from build123d import *

# Parameters (mm, degrees)
F0_W      = 25
F0_H      = 11
F1_DEPTH  = 10
F2_R      = 8
F3_DEPTH  = 6
F4_R      = 6
F5_DEPTH  = 4.2
F6_W      = 11
F6_H      = 10
F7_DEPTH  = 2
F8_W      = 11
F8_H      = 10
F9_DEPTH  = 2
F10_R     = 5
F11_R     = 1.75
F12_DEPTH = 25
F9_FACE_W = 19
F9_FACE_H = 10
F13_DEPTH = 10
F14_R     = 8.137493
F15_DEPTH = 4.5
F17_DEPTH = 7
F18_R     = 4.5
F19_DEPTH = 25


with BuildPart() as f1:
    # F0 (on Top) → F1 (new body)
    with BuildSketch(Plane.XY):
        with Locations((12.5, 5.5)):
            Rectangle(F0_W, F0_H)
    extrude(amount=F1_DEPTH)

    # F2 (on face) → F3 (cut)
    with BuildSketch(Plane.XZ):
        with Locations((12.5, 10)):
            Circle(F2_R)
    extrude(amount=-F3_DEPTH, mode=Mode.SUBTRACT)

    # F4 (on face) → F5 (cut)
    with BuildSketch(Plane.XZ.offset(-6)):
        with Locations((12.5, 10)):
            Circle(F4_R)
    extrude(amount=-F5_DEPTH, mode=Mode.SUBTRACT)

    # F6 (on face) → F7 (join)
    with BuildSketch(Plane(origin=(0, 0, 0), x_dir=(0, -1, 0), z_dir=(-1, 0, 0))):
        with Locations((-5.5, 5)):
            Rectangle(F6_W, F6_H)
    extrude(amount=F7_DEPTH)

    # F8 (on face) → F9 (join)
    with BuildSketch(Plane.YZ.offset(25)):
        with Locations((5.5, 5)):
            Rectangle(F8_W, F8_H)
    extrude(amount=F9_DEPTH)

    # F10
    f10_edges = [f1.edges().sort_by_distance(p)[0] for p in [
        (27, 11, 5),
        (27, 0, 5),
        (-2, 11, 5),
        (-2, 0, 5),
    ]]
    fillet(f10_edges, radius=F10_R)

    # F11 (on face) → F12 (cut)
    with BuildSketch(Plane.XY.offset(10)):
        with Locations((0.75, 6.25)):
            Circle(F11_R)
        with Locations((24.25, 6.25)):
            Circle(F11_R)
    extrude(amount=-F12_DEPTH, mode=Mode.SUBTRACT)

    # F9_face (on face) → F13 (join)
    with BuildSketch(Plane(origin=(12.5, 11, 5), x_dir=(-1, 0, 0), z_dir=(0, 1, 0))):
        Rectangle(F9_FACE_W, F9_FACE_H)
    extrude(amount=F13_DEPTH)

    # F14 (on face) → F15 (cut)
    with BuildSketch(Plane.XZ.offset(-10.2)):
        with Locations((12.5, 10)):
            Circle(F14_R)
    extrude(amount=-F15_DEPTH, mode=Mode.SUBTRACT)

    # F16 (on face) → F17 (join)
    with BuildSketch(Plane.XY.offset(10)):
        Polygon((3, 16.541481), (4.362507, 14.7), (20.637493, 14.7), (22, 16), (22, 21), (3, 21), align=None)
    extrude(amount=F17_DEPTH)

    # F18 (on face) → F19 (cut)
    with BuildSketch(Plane.XZ.offset(-14.7)):
        with Locations((12.5, 10)):
            Circle(F18_R)
    extrude(amount=-F19_DEPTH, mode=Mode.SUBTRACT)


solid = f1.part
The listing builds one solid part. Answer for the finished solid, in the listing's coordinates (mm). A direction names the side the tool comes from. Give positions to 0.01 mm unless a question says otherwise; leave off trailing zeros. Write each loop counter-clockwise with the first axis right and the second up, starting at its lowest first coordinate (ties: lowest second). Pieces come first, ordered by that corner, then holes. Notation, with made-up numbers: (6.25, 14.25) -> (48.25, 14.25) arc R32 ccw to (48.25, 41.25) -> close; hole circle Ø6 at (80, 20). An arc over 180 degrees is marked (long way). One line per question, with ' | ' between items. Start each with the question number.
1. Find the intervals of material crossed by probe 1 along Y at (x, z) = (19, 5.5); probe 2 along X at (y, z) = (5.75, 8); probe 3 along Z at (x, y) = (12.5, 18), in increasing order.
2. Section D-D (y = 2) is taken. Determine the outline of the cut face in (x, z).
3. Given pin 1 Ø3 at (y, z) = (14, 8) entering from +X; pin 2 Ø1 at (y, z) = (4, 2.5) entering from +X; pin 3 Ø2.5 at (x, y) = (1, 11) entering from +Z, each flat-ended and moving along its own axis, determine where each tip first touches the part or whether it passes through.
4. Section C-C (z = 11.5) is taken. Determine the outline of the cut face in (x, y).
5. Section A-A (x = 12.5) is taken. Determine the outline of the cut face in (y, z).
6. For faces 4 (the flat face through (21.31, 15.34, 13.45)), 5 (the cylindrical face through (12.321, 12.418, 1.864)), 6 (the flat face through (3.672, 15.634, 13.451)), 7 (the flat face through (22, 17, 6)), determine the directions among +Z, -Z, +X, -X, +Y, -Y from which every point of the face is accessible in a straight line to the end or side of a thin tool.
7. For a pull along X with two mould halves and no side action, classify faces 1 (the flat face through (3, 6, 10)), 2 (the cylindrical face through (12.324, 2.958, 2.002)), 3 (the cylindrical face through (25, 1, 5)) as pulls with the +X half, pulls with the -X half, needs draft (parallel to the pull), parting line crosses it, or undercut.
8. Section B-B (z = 9.5) is taken. Determine the outline of the cut face in (x, y), plus the area to 3 significant figures.
Response values:
1) probe 1: 6 to 10.2, 14.7 to 21 | probe 2: -2 to -0.93, 2.43 to 4.75, 20.25 to 22.57, 25.93 to 27 | probe 3: 0 to 5.5, 14.5 to 17
2) outline: (-1, 0) -> (26, 0) -> (26, 10) -> (20.5, 10) arc R8 cw to (4.5, 10) -> (-1, 10) -> close
3) pin 1: x = 22 | pin 2: x = 26.97 | pin 3: z = 10
4) outline: (3, 16.54) -> (4.36, 14.7) -> (8.26, 14.7) -> (8.26, 21) -> (3, 21) -> close; (16.74, 14.7) -> (20.64, 14.7) -> (22, 16) -> (22, 21) -> (16.74, 21) -> close
5) outline: (0, 0) -> (21, 0) -> (21, 5.5) -> (14.7, 5.5) -> (14.7, 1.86) -> (10.2, 1.86) -> (10.2, 4) -> (6, 4) -> (6, 2) -> (0, 2) -> close; (14.7, 14.5) -> (21, 14.5) -> (21, 17) -> (14.7, 17) -> close
6) face 4: +Z, +X, -Y | face 5: +Z | face 6: +Z, -X, -Y | face 7: +Z, -Z, +X, +Y
7) face 1: needs draft | face 2: undercut | face 3: pulls with the +X half
8) outline: (-2, 5) arc R5 ccw to (3, 0) -> (4.52, 0) -> (4.52, 6) -> (6.52, 6) -> (6.52, 10.2) -> (4.38, 10.2) -> (4.38, 14.7) -> (8.03, 14.7) -> (8.03, 21) -> (3, 21) -> (3, 11) arc R5 ccw to (-2, 6) -> close; (16.97, 14.7) -> (20.62, 14.7) -> (20.62, 10.2) -> (18.48, 10.2) -> (18.48, 6) -> (20.48, 6) -> (20.48, 0) -> (22, 0) arc R5 ccw to (27, 5) -> (27, 6) arc R5 ccw to (22, 11) -> (22, 21) -> (16.97, 21) -> close; hole circle Ø3.5 at (0.75, 6.25); hole circle Ø3.5 at (24.25, 6.25) | area: 193 mm2
